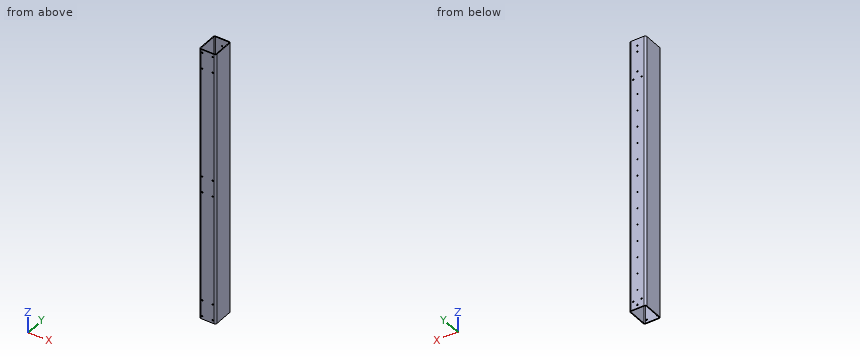
from build123d import *

# Parameters (mm, degrees)
BOSS_EXTRUDE1_DEPTH             = 990
TAP_DRILL_FOR_M6X1_0_TAP1_D     = 5
TAP_DRILL_FOR_M6X1_0_TAP1_DEPTH = 10
TAP_DRILL_FOR_M6X1_0_TAP1_TIP   = 1.502151548
TAP_DRILL_FOR_M5X0_8_TAP1_D     = 4.2
TAP_DRILL_FOR_M5X0_8_TAP1_DEPTH = 3
TAP_DRILL_FOR_M6X1_0_TAP2_D     = 5
TAP_DRILL_FOR_M6X1_0_TAP2_DEPTH = 3


with BuildPart() as part:
    # Sketch1 → Boss-Extrude1 (new body)
    with BuildSketch(Plane.XY):
        with BuildLine():
            Line((-30, -34), (-30, 34))
            ThreePointArc((-30, 34), (-28.242640687, 38.242640687), (-24, 40))
            Line((-24, 40), (24, 40))
            ThreePointArc((24, 40), (28.242640687, 38.242640687), (30, 34))
            Line((30, 34), (30, -34))
            ThreePointArc((30, -34), (28.242640687, -38.242640687), (24, -40))
            Line((24, -40), (-24, -40))
            ThreePointArc((-24, -40), (-28.242640687, -38.242640687), (-30, -34))
        make_face()
        with BuildLine():
            Line((-27, -34), (-27, 34))
            ThreePointArc((-27, 34), (-26.121320344, 36.121320344), (-24, 37))
            Line((-24, 37), (24, 37))
            ThreePointArc((24, 37), (26.121320344, 36.121320344), (27, 34))
            Line((27, 34), (27, -34))
            ThreePointArc((27, -34), (26.121320344, -36.121320344), (24, -37))
            Line((24, -37), (-24, -37))
            ThreePointArc((-24, -37), (-26.121320344, -36.121320344), (-27, -34))
        make_face(mode=Mode.SUBTRACT)
    extrude(amount=BOSS_EXTRUDE1_DEPTH)

    # Tap Drill for M6x1.0 Tap1
    with Locations(Plane(origin=(19, -40, 979), x_dir=(0, 0, -1), z_dir=(0, -1, 0))):
        with Locations((0, 0), (0, -38), (58, -38), (58, 0), (455, 0), (455, -38), (513, 0), (513, -38), (910, 0), (968, 0), (968, -38), (910, -38)):
            Hole(TAP_DRILL_FOR_M6X1_0_TAP1_D / 2, depth=TAP_DRILL_FOR_M6X1_0_TAP1_DEPTH)
            with Locations((0, 0, -(TAP_DRILL_FOR_M6X1_0_TAP1_DEPTH + TAP_DRILL_FOR_M6X1_0_TAP1_TIP / 2))):  # 118° drill point
                Cone(0, TAP_DRILL_FOR_M6X1_0_TAP1_D / 2, TAP_DRILL_FOR_M6X1_0_TAP1_TIP, mode=Mode.SUBTRACT)

    # Tap Drill for M5x0.8 Tap1
    with Locations(Plane(origin=(-0.018233765, 40, 787), x_dir=(0, 0, 1), z_dir=(0, 1, 0))):
        with Locations((0, 0), (-60, 0), (-120, 0), (-180, 0), (-240, 0), (-300, 0), (-360, 0), (-420, 0), (-480, 0), (-540, 0), (-600, 0), (-660, 0), (-720, 0)):
            Hole(TAP_DRILL_FOR_M5X0_8_TAP1_D / 2, depth=TAP_DRILL_FOR_M5X0_8_TAP1_DEPTH)

    # Tap Drill for M6x1.0 Tap2
    with Locations(Plane(origin=(0.15, 40, 965.5), x_dir=(0, 0, 1), z_dir=(0, 1, 0))):
        with Locations((0, 0), (-22.5, 0), (-95, 0), (-120, -15), (-120, 15), (-936.5, 15), (-953.5, 0), (-936.5, -15)):
            Hole(TAP_DRILL_FOR_M6X1_0_TAP2_D / 2, depth=TAP_DRILL_FOR_M6X1_0_TAP2_DEPTH)


solid = part.part
Build history of the part. All positions in model axes, mm. Give positions to 0.01 mm unless a question says otherwise; leave off trailing zeros. Order: outer loops, then holes, each group sorted by start corner. A loop starts at its lowest first (then second) coordinate and runs counter-clockwise, first axis right, second up. Notation, with made-up numbers: M 38,-24.75 L 61,-24.75 A17 cw 61,-8.75 Z; hole C 87.5,2.25 d3. An arc over 180 degrees is marked long. Put each result on its own line as item: value.
Item 1: Flat gauge pins, fed straight in: pin 1 Ø3.5 at (x, z) = (-0.02, 427) entering from +Y; pin 2 Ø5 at (x, y) = (-22.5, 18) entering from +Z. Where does each tip first touch, or does it go through?
From the geometry:
pin 1: stops at y = -37
pin 2: passes through
Item 2: Probe line 1 (Y direction, x = 24, z = 744); line 2 (X direction, y = 38.5, z = 29); line 3 (X direction, y = -0.5, z = 111.5). List the from-to ranges inside material, lowest first. Write a range as [from, to].
From the geometry:
line 1: y = [-40, -37], [37, 40]
line 2: x = [-27.97, -17.35], [-12.35, 12.65], [17.65, 27.97]
line 3: x = [-30, -27], [27, 30]
Item 3: Slice it at A-A, the plane y = -2. Write the cut outline in (x, z), plus the area to 3 significant figures.
From the geometry:
outline: M -30,0 L -27,0 L -27,990 L -30,990 Z; M 27,0 L 30,0 L 30,990 L 27,990 Z
area: 5,940 mm2
Item 4: Slice it at B-B, the plane z = 681.5. Write the cut outline in (x, y).
From the geometry:
outline: M -30,-34 A6 ccw -24,-40 L 24,-40 A6 ccw 30,-34 L 30,34 A6 ccw 24,40 L -24,40 A6 ccw -30,34 Z; hole M -27,-34 A3 ccw -24,-37 L 24,-37 A3 ccw 27,-34 L 27,34 A3 ccw 24,37 L -24,37 A3 ccw -27,34 Z
